from build123d import *

# Parameters (mm, degrees)
SKETCH027_W      = 4
SKETCH027_H      = 2.4
EXTRUDE024_DEPTH = 20
SKETCH_W         = 35
SKETCH_H         = 17
SKETCH_W_2       = 33
SKETCH_H_2       = 15
EXTRUDE_DEPTH    = 34


with BuildPart() as extrude024:
    # Sketch027 → Extrude024 (new body)
    with BuildSketch(Plane.XY.offset(18)):
        with Locations((25.5, -25.8)):
            Rectangle(SKETCH027_W, SKETCH027_H)
    extrude(amount=-EXTRUDE024_DEPTH)


with BuildPart() as cut001:
    # Sketch → Extrude (new body)
    with BuildSketch(Plane.XZ.offset(29)):
        with Locations((25.5, 7.5)):
            Rectangle(SKETCH_W, SKETCH_H)
        with Locations((25.5, 7.5)):
            Rectangle(SKETCH_W_2, SKETCH_H_2, mode=Mode.SUBTRACT)
    extrude(amount=-EXTRUDE_DEPTH)

    # Cut001: cut Extrude024
    add(extrude024.part, mode=Mode.SUBTRACT)


solid = cut001.part
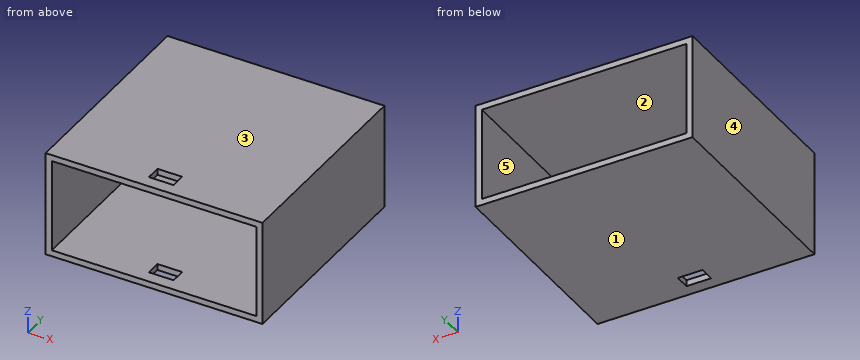
Here's how the part is built. I have some questions about the finished solid (model axes, mm). Face numbers are marked on the shaded views. A direction names the side the tool comes from. Give positions to 0.01 mm unless a question says otherwise; leave off trailing zeros. Write each loop counter-clockwise with the first axis right and the second up, starting at its lowest first coordinate (ties: lowest second). Pieces come first, ordered by that corner, then holes. Notation, with made-up numbers: (-24.5, -20) -> (4.5, -20) arc R17 cw to (4.5, -3) -> close; hole circle Ø11 at (22.5, -28). An arc over 180 degrees is marked (long way). Use one line per item in the form item = value. Start each with the question number.
1. Thinking about a two-plate mould opening in X: for the marked faces 3, 4 and 5, which applies, +X half, -X half, draft (parallel to the pull), parting line (faces both ways), or undercut?
2. Imagine slicing it at B-B on y = -13.5. List the corners of the cut face in (x, z) for me, plus the area to 3 significant figures.
3. If I drill on L1, parallel to Z at x = 20.5, y = -11; L2, parallel to X at y = -4.5, z = 3.5, over which ranges is the centre line in solid material (lowest first)?
4. Imagine slicing it at A-A on z = 7.5. List the corners of the cut face in (x, y) for me, plus the area to 3 significant figures.
5. Imagine slicing it at C-C on x = 34. List the corners of the cut face in (y, z) for me.
6. On a 3-axis mill with a long thin cutter (end or side, diameter ignored), from which of +Z, -Z, +X, -X, +Y, -Y can I reach the whole of each face in a straight line? I mean the marked faces 1 and 2. Say none if no direction works.
Entries:
q1.face_3 = draft
q1.face_4 = -X half
q1.face_5 = undercut
q2.outline = (8, -1) -> (43, -1) -> (43, 16) -> (8, 16) -> close; hole (9, 0) -> (42, 0) -> (42, 15) -> (9, 15) -> close
q2.area = 100 mm²
q3.L1 = -1 to 0, 15 to 16
q3.L2 = 8 to 9, 42 to 43
q4.outline = (8, -29) -> (9, -29) -> (9, 5) -> (8, 5) -> close; (42, -29) -> (43, -29) -> (43, 5) -> (42, 5) -> close
q4.area = 68.0 mm²
q5.outline = (-29, -1) -> (5, -1) -> (5, 0) -> (-29, 0) -> close; (-29, 15) -> (5, 15) -> (5, 16) -> (-29, 16) -> close
q6.face_1 = -Z, +X, -X, +Y, -Y
q6.face_2 = +Y, -Y
